Autodesk Inventor part; units mm, degrees
ref_plane "YZ Plane" through (0, 0, 0) normal (1, 0, 0) x (0, 1, 0)
ref_plane "XZ Plane" through (0, 0, 0) normal (0, 1, 0) x (-1, 0, 0)
ref_plane "XY Plane" through (0, 0, 0) normal (0, 0, 1) x (1, 0, 0)
sketch "Эскиз1" plane through (0, 0, 0) normal (0, 0, 1) x (1, 0, 0)
  line L0 (0, 0) -> (20, 0)
  line L1 (0, 0) -> (0, 12.5)
  line L2 (0, 12.5) -> (0, 16.5)
  line L3 (0, 12.5) -> (20, 12.5)
  line L4 (20, 0) -> (20, 15)
  line L5 (20, 15) -> (35, 15)
  line L6 (35, 15) -> (35, 0)
  line L7 (35, 0) -> (20, 0)
  line L8 (0, 16.5) -> (20, 16.5)
  line L9 (20, 15) -> (20, 16.5)
  dimension "d0" = 20
  dimension "d1" = 12.5
  dimension "d2" = 4
  dimension "d5" = 15
  dimension "d6" = 15
revolve "Вращение1" add sketch "Эскиз1" angle 360 about axis through (0, 0, 0) along (1, 0, 0) contours L4 L5 L6 L7 | L2 L8 L9 L4 L3
sketch "Эскиз2" plane through (0, 0, 0) normal (0, 0, 1) x (1, 0, 0)
  line L0 (0, 0) -> (10, 0)
  circle A0 centre (10, 0) radius 1.5
  dimension "d8" = 10
  dimension "d9" = 3
extrude "Выдавливание1" cut sketch "Эскиз2" along normal mid plane 40
thread "Резьба1"
sketch "Эскиз3" plane through (35, 0, 0) normal (1, 0, 0) x (0, 0, -1)
  line L0 (0, 0) -> (-5, 0)
  line L1 (-5, 0) -> (-5, 20)
  line L2 (-5, 20) -> (5, 20)
  line L3 (5, 20) -> (5, -20)
  line L4 (5, -20) -> (-5, -20)
  line L5 (-5, -20) -> (-5, 0)
  circle A0 centre (0, 0) radius 15
  line L6 (0, 0) -> (0, 5)
  line L7 (0, 5) -> (-20, 5)
  line L8 (-20, 5) -> (-20, -5)
  line L9 (-20, -5) -> (20, -5)
  line L10 (20, -5) -> (20, 5)
  line L11 (20, 5) -> (0, 5)
  point P0 (-5, -5)
  point P1 (-14.1421, -5)
  point P2 (-5, -14.1421)
  point P3 (14.1421, -5)
  point P4 (5, -5)
  point P5 (5, -14.1421)
  point P6 (5, 5)
  point P7 (14.1421, 5)
  point P8 (5, 14.1421)
  point P9 (-14.1421, 5)
  point P10 (-5, 5)
  point P11 (-5, 14.1421)
  dimension "d14" = 5
  dimension "d15" = 10
  dimension "d16" = 5
  dimension "d17" = 10
extrude "Выдавливание2" cut sketch "Эскиз3" against normal blind 10 contours L7 A0 L1 | L5 A0 L9 | L3 A0 L11 | L9 A0 L3
properties part number "Втулка двигатель, вал"
Work out the finished part from the listing and answer in its coordinate system (mm). A direction names the side the tool comes from. Give positions to 0.01 mm unless a question says otherwise; leave off trailing zeros. Loops run counter-clockwise (first coordinate to the right, second up) from the corner with the lowest first, then second, coordinate; pieces in that order, holes last. Notation, with made-up numbers: M 34.5,57 L 51.5,57 A16 ccw 51.5,72 Z; hole C 65,64.5 d7. An arc over 180 degrees is marked long. Use CSV: the item, a comma, the result in double quotes.
1) Which of the six approach directions +Z, -Z, +X, -X, +Y, -Y give full straight-line access (tool end or side, diameter ignored) to faces 4 (the flat face through (30, 10, 5)), 5 (the cylindrical face through (24.272, -11.056, 10.138)), 6 (the flat face through (30, -10, 5))?
Answer:
face 4,"+Z, +X, +Y"
face 5,"+X"
face 6,"+Z, +X, -Y"
2) Determine the mould class of faces 1 (the flat face through (20, 4, -15)), 2 (the flat face through (30, -10, -5)), 3 (the cylindrical face through (8.5, 0.07, -14.43)) for opening direction X: released by +X, released by -X, zero draft, split by the parting line, or undercut.
Answer:
face 1,"released by +X"
face 2,"zero draft"
face 3,"undercut"
3) Given P1, Ø10, axis at x = 29.5, y = 7, coming from the -Z side; P2, Ø2.5, axis at x = 10, y = 0, coming from the -Z side; P3, Ø2.5, axis at x = 32, z = 10.5, coming from the -Y side; P4, Ø6, axis at x = 25, z = -2.5, coming from the +Y side, each flat-ended and moving along its own axis, determine where each tip first touches the part or whether it passes through.
Answer:
P1,"z = -14.87"
P2,"through"
P3,"y = -5"
P4,"y = 15"
4) Find section B-B on x = 26. Write down the section's boundary in (y, z).
Answer:
outline,"M -14.14,-5 L -5,-5 L -5,-14.14 A15 ccw 5,-14.14 L 5,-5 L 14.14,-5 A15 ccw 14.14,5 L 5,5 L 5,14.14 A15 ccw -5,14.14 L -5,5 L -14.14,5 A15 ccw Z"
5) Find section D-D on z = 0. Write down the section's boundary in (x, y), plus the area to 3 significant figures.
Answer:
outline,"M 0,-16.5 L 20,-16.5 L 20,-15 L 35,-15 L 35,15 L 20,15 L 20,16.5 L 0,16.5 L 0,12.5 L 20,12.5 L 20,-12.5 L 0,-12.5 Z"
area,"610 mm^2"
6) Find section C-C on z = -13.5. Write down the section's boundary in (x, y).
Answer:
outline,"M 0,-9.49 L 20,-9.49 L 20,-6.54 L 25,-6.54 L 25,-5 L 35,-5 L 35,5 L 25,5 L 25,6.54 L 20,6.54 L 20,9.49 L 0,9.49 Z; hole C 10,0 d3"
7) Find section A-A on y = 0. Write down the section's boundary in (x, z), plus the area to 3 significant figures.
Answer:
outline,"M 0,-16.5 L 8.5,-16.5 L 8.5,-12.5 L 0,-12.5 Z; M 0,12.5 L 8.5,12.5 L 8.5,16.5 L 0,16.5 Z; M 11.5,-16.5 L 20,-16.5 L 20,-15 L 35,-15 L 35,15 L 20,15 L 20,16.5 L 11.5,16.5 L 11.5,12.5 L 20,12.5 L 20,-12.5 L 11.5,-12.5 Z"
area,"586 mm^2"
8) Consider L1, parallel to X at y = 0, z = -14.65; L2, parallel to Z at x = 6.75, y = 0; L3, parallel to X at y = -11.5, z = -10. Determine where each line is inside the solid, lowest interval first.
Answer:
L1,"0 to 8.5, 11.5 to 35"
L2,"-16.5 to -12.5, 12.5 to 16.5"
L3,"0 to 20"
